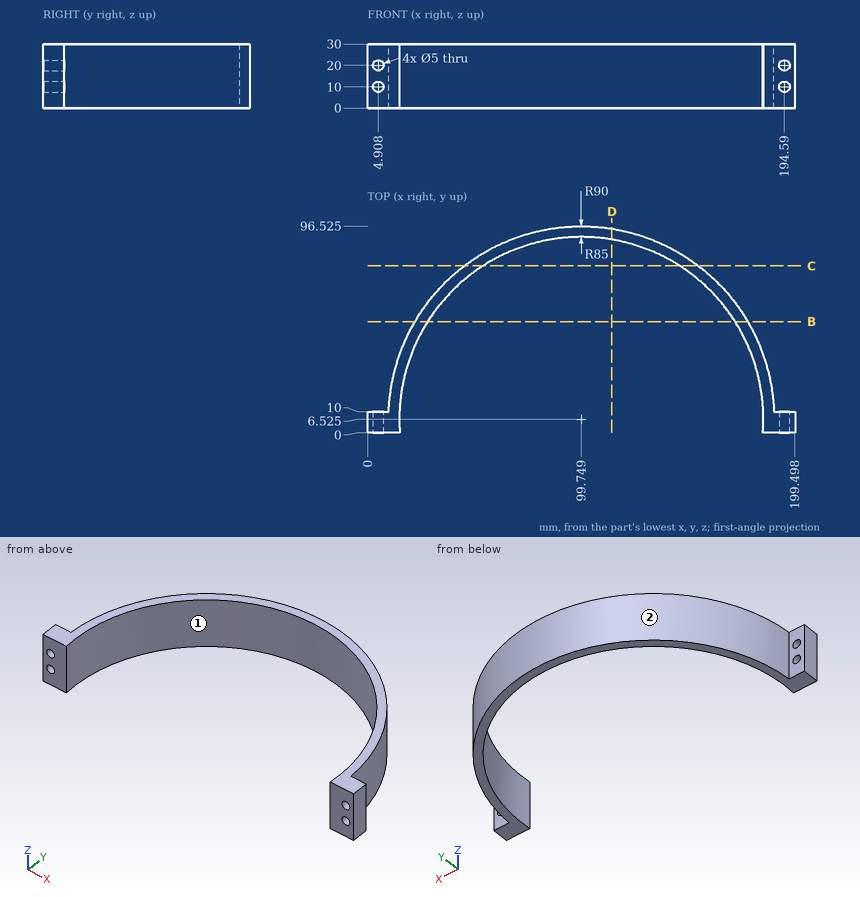
For this review, use the dimensioned drawing (mm, ordinates from the lowest corner) and the shaded views. Give positions to 0.01 mm unless a question says otherwise; leave off trailing zeros. Write each loop counter-clockwise with the first axis right and the second up, starting at its lowest first coordinate (ties: lowest second). Pieces come first, ordered by that corner, then holes. Notation, with made-up numbers: M 9.5,-38 L 13.5,-38 A19 cw 13.5,-9 Z; hole C 72,4 d5. An arc over 180 degrees is marked long. Answer as a JSON object with one key per item and string values. Group by question number.
Item 1: For pin 1 Ø1 at (x, z) = (108, 25.5) entering from -Y; pin 2 Ø8 at (x, z) = (156, 11.5) entering from +Y (1 decimal); pin 3 Ø8 at (x, z) = (66, 7) entering from +Y, all flat-tipped, find the tip position at first contact; note any pin that passes through.
Item 2: Consider section D-D on x = 114. Write out the cut boundary in (y, z), plus the area to 3 significant figures.
Item 3: Draft analysis for pull direction X (two halves, no side actions). For the marked faces 1 and 2, state which applies: +X half, -X half, draft (parallel to the pull), parting line (faces both ways), or undercut.
Item 4: For probe 1 along X at (y, z) = (7.5, 3.5) (1 decimal); probe 2 along X at (y, z) = (76, 25.25) (1 decimal); probe 3 along Y at (x, z) = (28.5, 18.5) (1 decimal), list the stretches that pass through material, from the lowest coordinate up. Write a range as [from, to].
Item 5: Consider section C-C on y = 78. Write out the cut boundary in (x, z) (1 decimal).
Item 6: Consider section B-B on y = 52. Write out the cut boundary in (x, z) (1 decimal), plus the area to 3 significant figures.
Check result:
{
 "1": {"pin 1": "stops at y = 91.07", "pin 2": "stops at y = 79.8", "pin 3": "stops at y = 91.47"},
 "2": {"outline": "M 90.32,0 L 95.39,0 L 95.39,30 L 90.32,30 Z", "area": "152 mm^2"},
 "3": {"face 1": "undercut", "face 2": "parting line"},
 "4": {"probe 1": "x = [0, 14.8], [184.7, 199.5]", "probe 2": "x = [42.5, 50.8], [148.7, 157]", "probe 3": "y = [52.9, 61.5]"},
 "5": {"outline": "M 45.1,0 L 53.7,0 L 53.7,30 L 45.1,30 Z; M 145.8,0 L 154.4,0 L 154.4,30 L 145.8,30 Z"},
 "6": {"outline": "M 22.1,0 L 27.9,0 L 27.9,30 L 22.1,30 Z; M 171.6,0 L 177.4,0 L 177.4,30 L 171.6,30 Z", "area": "351 mm^2"}
}
